Check sheet for the modelled part. Datum: model origin and axes. Units: mm. A direction names the side the tool comes from. Give positions to 0.01 mm unless a question says otherwise; leave off trailing zeros. Order: outer loops, then holes, each group sorted by start corner. A loop starts at its lowest first (then second) coordinate and runs counter-clockwise, first axis right, second up.
Item 1: Sectioned sample at B-B on x = 29. Record the boundary of the cut face in (y, z).
Item 2: Access from +Z, -Z, +X, -X, +Y, -Y to the whole of each face (thin tool, end or side, straight path). Record for faces 3 (the cylindrical face through (1.521, 61.8, -13.498)), 4 (the flat face through (55, 35, -12)).
Item 3: Sectioned sample at D-D on z = -4. Record the boundary of the cut face in (x, y), and give its area (3 significant figures).
Item 4: Material ranges on line 1 along Y through (x, z) = (55.65, -12.5); line 2 along X through (y, z) = (2.4, -8.5); line 3 along X through (y, z) = (21.5, -19), recorded low to high.
Item 5: Gauge pin test, flat ends, axial feed: P1, Ø2.5, axis at x = 24.5, z = -8.5, coming from the -Y side; P2, Ø5, axis at x = 23, z = -8, coming from the +Y side; P3, Ø6.5, axis at y = 55.5, z = -12.5, coming from the -X side. Record the tip position at first contact, or that the pin passes through.
Item 6: Sectioned sample at C-C on y = 61.5. Record the boundary of the cut face in (x, z).
Item 7: Release check for a two-part mould opening along Z. For faces 1 (the flat face through (29, 0, -18)), 2 (the cylindrical face through (56.48, 56.49, -6.41)) record: released by +Z, released by -Z, zero draft, split by the parting line, or undercut.
Item 8: Sectioned sample at A-A on y = 26.5. Record the boundary of the cut face in (x, z).
from build123d import *

# Parameters (mm, degrees)
SKETCH1_W               = 58
SKETCH1_H               = 25
BOSS_EXTRUDE1_DEPTH     = 3
SKETCH2_W               = 3
SKETCH2_H               = 25
BOSS_EXTRUDE2_DEPTH     = 65
CUT_EXTRUDE1_DEPTH      = 65
SKETCH4_R               = 4
CUT_EXTRUDE2_DEPTH      = 65
SKETCH5_R               = 1
CUT_EXTRUDE3_DEPTH      = 56
CUT_EXTRUDE3_DEPTH_BACK = 4
CUT_EXTRUDE5_REACH      = 70
SKETCH7_R               = 4
SKETCH7_R_2             = 1


with BuildPart() as part:
    # Sketch1 → Boss-Extrude1 (new body)
    with BuildSketch(Plane(origin=(0, 0, 0), x_dir=(1, 0, 0), z_dir=(0, 1, 0))):
        with Locations((29, 12.5)):
            Rectangle(SKETCH1_W, SKETCH1_H)
    extrude(amount=BOSS_EXTRUDE1_DEPTH)

    # Sketch2 → Boss-Extrude2 (add)
    with BuildSketch(Plane(origin=(0, 3, 0), x_dir=(1, 0, 0), z_dir=(0, 1, 0))):
        with Locations((56.5, 12.5)):
            Rectangle(SKETCH2_W, SKETCH2_H)
        with Locations((1.5, 12.5)):
            Rectangle(SKETCH2_W, SKETCH2_H)
    extrude(amount=BOSS_EXTRUDE2_DEPTH)

    # Sketch3 → Cut-Extrude1 (cut)
    with BuildSketch(Plane.ZY):
        with BuildLine():
            Line((-25, 68), (-25, 55.5))
            ThreePointArc((-25, 55.5), (-21.338834765, 64.338834765), (-12.5, 68))
            Line((-12.5, 68), (-25, 68))
        make_face()
        with BuildLine():
            Line((0, 68), (-12.5, 68))
            ThreePointArc((-12.5, 68), (-3.661165235, 64.338834765), (0, 55.5))
            Line((0, 55.5), (0, 68))
        make_face()
    extrude(amount=-CUT_EXTRUDE1_DEPTH, mode=Mode.SUBTRACT)

    # Sketch4 → Cut-Extrude2 (cut)
    with BuildSketch(Plane.ZY):
        with Locations((-12.5, 55.5)):
            Circle(SKETCH4_R)
    extrude(amount=-CUT_EXTRUDE2_DEPTH, mode=Mode.SUBTRACT)

    # Sketch5 → Cut-Extrude3 (cut, two sides)
    with BuildSketch(Plane(origin=(3, 0, 0), x_dir=(0, 0, -1), z_dir=(1, 0, 0))) as cut_extrude3_sk:
        with Locations((12.543720091, 61.500000009)):
            Circle(SKETCH5_R)
        with Locations((18.543720091, 55.500000009)):
            Circle(SKETCH5_R)
        with Locations((6.543720091, 55.500000009)):
            Circle(SKETCH5_R)
        with Locations((12.543720091, 49.500000009)):
            Circle(SKETCH5_R)
    extrude(amount=CUT_EXTRUDE3_DEPTH, mode=Mode.SUBTRACT)
    extrude(cut_extrude3_sk.sketch, amount=-CUT_EXTRUDE3_DEPTH_BACK, mode=Mode.SUBTRACT)

    # Sketch7 → Cut-Extrude5 (cut, up to next)
    with BuildSketch(Plane(origin=(0, 0, 0), x_dir=(-1, 0, 0), z_dir=(0, -1, 0)), mode=Mode.PRIVATE) as cut_extrude5_sk1:
        with Locations((-29, 13)):
            Circle(SKETCH7_R)
    cut_extrude5_tool1 = extrude(cut_extrude5_sk1.sketch, amount=-CUT_EXTRUDE5_REACH, mode=Mode.PRIVATE) & part.part
    add(cut_extrude5_tool1.solids().sort_by_distance((29, 0, -13))[0], mode=Mode.SUBTRACT)
    # Sketch7 → Cut-Extrude5 (cut, up to next)
    with BuildSketch(Plane(origin=(0, 0, 0), x_dir=(-1, 0, 0), z_dir=(0, -1, 0)), mode=Mode.PRIVATE) as cut_extrude5_sk2:
        with Locations((-24.5, 17.5)):
            Circle(SKETCH7_R_2)
    cut_extrude5_tool2 = extrude(cut_extrude5_sk2.sketch, amount=-CUT_EXTRUDE5_REACH, mode=Mode.PRIVATE) & part.part
    add(cut_extrude5_tool2.solids().sort_by_distance((24.5, 0, -17.5))[0], mode=Mode.SUBTRACT)
    # Sketch7 → Cut-Extrude5 (cut, up to next)
    with BuildSketch(Plane(origin=(0, 0, 0), x_dir=(-1, 0, 0), z_dir=(0, -1, 0)), mode=Mode.PRIVATE) as cut_extrude5_sk3:
        with Locations((-33.5, 17.5)):
            Circle(SKETCH7_R_2)
    cut_extrude5_tool3 = extrude(cut_extrude5_sk3.sketch, amount=-CUT_EXTRUDE5_REACH, mode=Mode.PRIVATE) & part.part
    add(cut_extrude5_tool3.solids().sort_by_distance((33.5, 0, -17.5))[0], mode=Mode.SUBTRACT)
    # Sketch7 → Cut-Extrude5 (cut, up to next)
    with BuildSketch(Plane(origin=(0, 0, 0), x_dir=(-1, 0, 0), z_dir=(0, -1, 0)), mode=Mode.PRIVATE) as cut_extrude5_sk4:
        with Locations((-33.5, 8.5)):
            Circle(SKETCH7_R_2)
    cut_extrude5_tool4 = extrude(cut_extrude5_sk4.sketch, amount=-CUT_EXTRUDE5_REACH, mode=Mode.PRIVATE) & part.part
    add(cut_extrude5_tool4.solids().sort_by_distance((33.5, 0, -8.5))[0], mode=Mode.SUBTRACT)
    # Sketch7 → Cut-Extrude5 (cut, up to next)
    with BuildSketch(Plane(origin=(0, 0, 0), x_dir=(-1, 0, 0), z_dir=(0, -1, 0)), mode=Mode.PRIVATE) as cut_extrude5_sk5:
        with Locations((-24.5, 8.5)):
            Circle(SKETCH7_R_2)
    cut_extrude5_tool5 = extrude(cut_extrude5_sk5.sketch, amount=-CUT_EXTRUDE5_REACH, mode=Mode.PRIVATE) & part.part
    add(cut_extrude5_tool5.solids().sort_by_distance((24.5, 0, -8.5))[0], mode=Mode.SUBTRACT)


solid = part.part
Report:
1. outline: (0, -25) - (3, -25) - (3, -17) - (0, -17) - close; (0, -9) - (3, -9) - (3, 0) - (0, 0) - close
2. face 3: +X, -X
2. face 4: +Z, -Z, +Y
3. outline: (0, 0) - (58, 0) - (58, 64.67) - (55, 64.67) - (55, 3) - (3, 3) - (3, 64.67) - (0, 64.67) - close
3. area: 544 mm2
4. line 1: y = 0 to 48.5, 50.5 to 51.5, 59.5 to 60.5, 62.5 to 68
4. line 2: x = 0 to 23.5, 25.5 to 32.5, 34.5 to 58
4. line 3: x = 0 to 3, 55 to 58
5. P1: stops at y = 0
5. P2: stops at y = 3
5. P3: passes through
6. outline: (0, -23.47) - (3, -23.47) - (3, -13.54) - (0, -13.54) - close; (0, -11.54) - (3, -11.54) - (3, -1.53) - (0, -1.53) - close; (55, -23.47) - (58, -23.47) - (58, -13.54) - (55, -13.54) - close; (55, -11.54) - (58, -11.54) - (58, -1.53) - (55, -1.53) - close
7. face 1: zero draft
7. face 2: undercut
8. outline: (0, -25) - (3, -25) - (3, 0) - (0, 0) - close; (55, -25) - (58, -25) - (58, 0) - (55, 0) - close
